from build123d import *

# Parameters (mm, degrees)
F0_W     = 25.4
F0_H     = 6.35
F1_ANGLE = 100.914843


with BuildPart() as f1:
    # F0 (on Right) → F1 (revolve, symmetric)
    with BuildSketch(Plane.YZ) as f1_sk:
        with Locations((12.7, 3.175)):
            Rectangle(F0_W, F0_H)
        Polygon((-7.733337, 0), (0, 0), (0, 6.35), (0, 13.47493), (-7.733337, 13.47493), align=None)
        Polygon((25.4, 6.35), (25.4, 0), (32.637283, 0), (32.637283, 13.47493), (25.4, 13.47493), align=None)
    revolve(axis=Axis((0, 12.517576, 101.6), (0, 1, 0)), revolution_arc=F1_ANGLE / 2)
    revolve(f1_sk.sketch, axis=Axis((0, 12.517576, 101.6), (0, -1, 0)), revolution_arc=F1_ANGLE / 2)


solid = f1.part
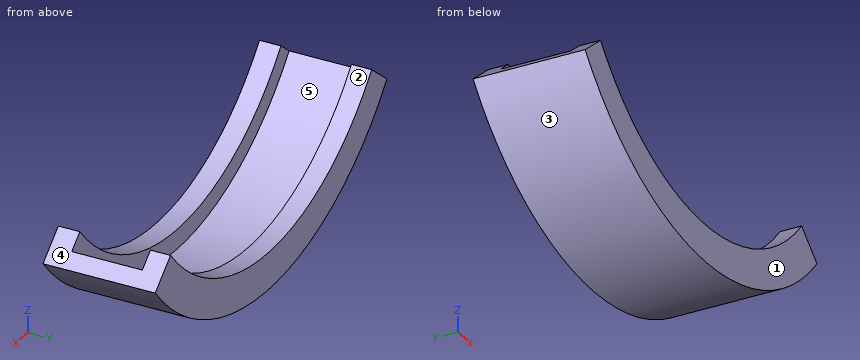
Work out the finished part from the listing and answer in its coordinate system (mm). Face numbers are marked on the shaded views. A direction names the side the tool comes from. Round coordinates to 2 decimals unless told otherwise and drop trailing zeros. Loops run counter-clockwise (first coordinate to the right, second up) from the corner with the lowest first, then second, coordinate; pieces in that order, holes last. Notation, with made-up numbers: M 9.5,2.5 L 58.5,2.5 A8 cw 58.5,8.5 Z; hole C -23,-15 d11. An arc over 180 degrees is marked long. One line per question, with ' | ' between items. Start each with the question number.
(1) A cutting plane is placed at D-D on z = 20. Write down the section's boundary in (x, y).
(2) A cutting plane is placed at B-B on x = -45. Write down the section's boundary in (y, z).
(3) A cutting plane is placed at A-A on z = 31. Write down the section's boundary in (x, y).
(4) Find the intervals of material crossed by line 1 (Y direction, x = 59.5, z = 27.5); line 2 (X direction, y = -1, z = 24); line 3 (X direction, y = 8.5, z = 31), in increasing order.
(5) Flat-ended cylindrical pins translate along their axes: pin 1 Ø1.5 at (y, z) = (25, 27) entering from +X; pin 2 Ø2 at (y, z) = (13.5, 16.5) entering from -X; pin 3 Ø1.5 at (x, y) = (-50, 26) entering from -Z; pin 4 Ø10 at (y, z) = (7.5, 32) entering from +X. Find the tip coordinate at first contact, or state that the pin passes through.
(6) A cutting plane is placed at C-C on y = -2.5. Write down the section's boundary in (x, z).
(7) A tool of negligible diameter and unlimited length cuts with its end or side. For the marked faces 4 and 5, from which of +Z, -Z, +X, -X, +Y, -Y can it reach the whole face along a straight path? Write none if from no direction.
(8) For a pull along X with two mould halves and no side action, classify the marked faces 1, 2 and 3 as released by +X, released by -X, zero draft, split by the parting line, or undercut.
Geometry check:
1) outline: M -60.53,-7.73 L -33.28,-7.73 L -33.28,0 L -49.13,0 L -49.13,25.4 L -33.28,25.4 L -33.28,32.64 L -60.53,32.64 Z; M 33.28,-7.73 L 60.53,-7.73 L 60.53,32.64 L 33.28,32.64 L 33.28,25.4 L 49.13,25.4 L 49.13,0 L 33.28,0 Z
2) outline: M -7.73,10.51 L 32.64,10.51 L 32.64,25.83 L 25.4,25.83 L 25.4,17.65 L 0,17.65 L 0,25.83 L -7.73,25.83 Z
3) outline: M -73.06,-7.73 L -52.74,-7.73 L -52.74,0 L -63.94,0 L -63.94,25.4 L -52.74,25.4 L -52.74,32.64 L -73.06,32.64 Z; M 52.74,-7.73 L 73.06,-7.73 L 73.06,32.64 L 52.74,32.64 L 52.74,25.4 L 63.94,25.4 L 63.94,0 L 52.74,0 Z
4) line 1: y = -7.73 to 0, 25.4 to 32.64 | line 2: x = -65.58 to -41.76, 41.76 to 65.58 | line 3: x = -73.06 to -63.94, 63.94 to 73.06
5) pin 1: stops at x = 69.78 | pin 2: stops at x = -57.01 | pin 3: stops at z = 12.73 | pin 4: stops at x = 78.35
6) outline: M -78.35,36.92 A101.6 ccw 78.35,36.92 L 67.96,45.5 A88.13 cw -67.96,45.5 Z
7) face 4: +Z, +X, +Y, -Y | face 5: +Z
8) face 1: zero draft | face 2: undercut | face 3: split by the parting line
